```python
from build123d import *

# Parameters (mm, degrees)
SKETCH1_R           = 2.5
BOSS_EXTRUDE1_DEPTH = 38
SKETCH2_R           = 10
SKETCH2_R_2         = 2
CUT_EXTRUDE1_DEPTH  = 38


with BuildPart() as part:
    # Sketch1 → Boss-Extrude1 (new body)
    with BuildSketch(Plane.XY):
        Polygon((-30, 0), (-30, -9), (-21, -9), (-21, -4), (21, -4), (21, -9), (30, -9), (30, 0), align=None)
        with Locations((-25.5, -4.5)):
            Circle(SKETCH1_R, mode=Mode.SUBTRACT)
        with Locations((25.5, -4.5)):
            Circle(SKETCH1_R, mode=Mode.SUBTRACT)
    extrude(amount=BOSS_EXTRUDE1_DEPTH)

    # Sketch2 → Cut-Extrude1 (cut)
    with BuildSketch(Plane.XZ.offset(4)):
        with Locations((0, 19)):
            Circle(SKETCH2_R)
        with Locations((0, 33.5)):
            Circle(SKETCH2_R_2)
        with Locations((12.557368355, 11.75)):
            Circle(SKETCH2_R_2)
        with Locations((-12.557368355, 11.75)):
            Circle(SKETCH2_R_2)
    extrude(amount=-CUT_EXTRUDE1_DEPTH, mode=Mode.SUBTRACT)


solid = part.part
```
Geometry check sheet. Reference: the model listing, model coordinates, mm. A direction names the side the tool comes from. Round coordinates to 2 decimals unless told otherwise and drop trailing zeros. Loops run counter-clockwise (first coordinate to the right, second up) from the corner with the lowest first, then second, coordinate; pieces in that order, holes last. Notation, with made-up numbers: (-6.5, -37) - (42.5, -37) arc R11 cw to (42.5, -26) - close; hole circle Ø5 at (32, -25.75). An arc over 180 degrees is marked (long way). Write item = value, one per line. Start each with the question number.
1. Depth check by flat-ended pin: pin 1 (1 mm diameter, centred on x = -22.5, y = -6.5, fed in from -Z); pin 2 (1 mm diameter, centred on x = 10, z = 28, fed in from -Y). Enter the tip coordinate at first touch or a pass-through.
2. Section check B-B on z = 19. Enter the section's corners in (x, y).
3. Section check D-D on z = 6. Enter the section's corners in (x, y).
4. Thickness scan on line 1 (Z direction, x = 0, y = -2.35); line 2 (X direction, y = -8.25, z = 21.5); line 3 (X direction, y = -5.25, z = 24). Record the ranges inside material, lowest first.
5. Set-up check for faces 4 (the face through (21, -6, 19)), 5 (the face through (30, -5, 19)): record each of +Z, -Z, +X, -X, +Y, -Y from which the full face is reachable in a straight line by a thin tool's end or side.
6. Section check A-A on x = -8. Enter the section's corners in (y, z), then the cut area to 3 significant figures.
7. Section check C-C on x = 0. Enter the section's corners in (y, z).
8. Mould release check, pull along Z, two halves, no side actions. Record for faces 1 (the face through (-28, -4.4, 18.7)), 2 (the face through (0, -2, 38)), 3 (the face through (-14.555, -2.028, 11.838)): released by +Z, released by -Z, zero draft, split by the parting line, or undercut.
Working result:
q1.pin_1 = 0
q1.pin_2 = -4
q2.outline = (-30, -9) - (-21, -9) - (-21, -4) - (-10, -4) - (-10, 0) - (-30, 0) - close; (10, -4) - (21, -4) - (21, -9) - (30, -9) - (30, 0) - (10, 0) - close; hole circle Ø5 at (-25.5, -4.5); hole circle Ø5 at (25.5, -4.5)
q3.outline = (-30, -9) - (-21, -9) - (-21, -4) - (21, -4) - (21, -9) - (30, -9) - (30, 0) - (-30, 0) - close; hole circle Ø5 at (-25.5, -4.5); hole circle Ø5 at (25.5, -4.5)
q4.line_1 = 0 to 9, 29 to 31.5, 35.5 to 38
q4.line_2 = -30 to -21, 21 to 30
q4.line_3 = -30 to -27.88, -23.12 to -21, 21 to 23.12, 27.88 to 30
q5.face_4 = +Z, -Z, -Y
q5.face_5 = +Z, -Z, +X, +Y, -Y
q6.outline = (-4, 0) - (0, 0) - (0, 13) - (-4, 13) - close; (-4, 25) - (0, 25) - (0, 38) - (-4, 38) - close
q6.area = 104 mm^2
q7.outline = (-4, 0) - (0, 0) - (0, 9) - (-4, 9) - close; (-4, 29) - (0, 29) - (0, 31.5) - (-4, 31.5) - close; (-4, 35.5) - (0, 35.5) - (0, 38) - (-4, 38) - close
q8.face_1 = zero draft
q8.face_2 = released by +Z
q8.face_3 = undercut
